Could you check a few things on this drawing? It's one solid part, dimensions in mm from its lowest x, y, z. A direction names the side the tool comes from. Round coordinates to 2 decimals unless told otherwise and drop trailing zeros. Loops run counter-clockwise (first coordinate to the right, second up) from the corner with the lowest first, then second, coordinate; pieces in that order, holes last. Notation, with made-up numbers: (79, 16) -> (106, 16) arc R27 cw to (106, 54) -> close; hole circle Ø5 at (83.25, 30.5). An arc over 180 degrees is marked (long way). Write each question's results on one line, items separated by ' | '.
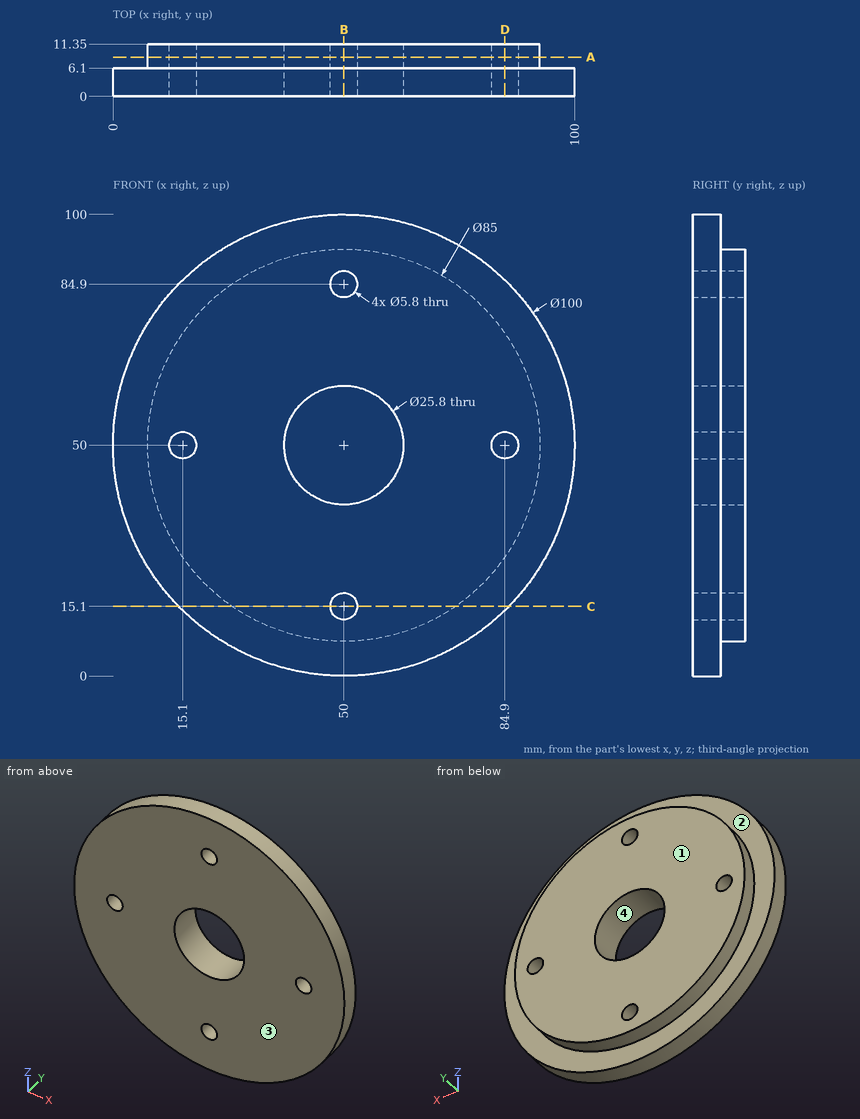
1) I need wall thicknesses on line 1 (X direction, y = 6.25, z = 50); line 2 (Z direction, x = 50, y = 4.5). Which ranges of each line are inside material? Lowest first, please.
Model answer:
line 1: x = 7.5 to 12.2, 18 to 37.1, 62.9 to 82, 87.8 to 92.5 | line 2: z = 0 to 12.2, 18 to 37.1, 62.9 to 82, 87.8 to 100
2) I'm going to push flat-ended pins straight in: pin 1 (3 mm diameter, centred on x = 40.5, z = 52.5, fed in from -Y); pin 2 (2 mm diameter, centred on x = 33.5, z = 51, fed in from -Y); pin 3 (2 mm diameter, centred on y = 2, z = 18.5, fed in from -X); pin 4 (6 mm diameter, centred on x = 38.5, y = 8.5, fed in from -Z). Where does each tip first touch, or does it pass through?
Model answer:
pin 1: passes through | pin 2: stops at y = 0 | pin 3: stops at x = 10.38 | pin 4: stops at z = 0.95
3) I want a section at C-C, the plane z = 15.1. Write out the boundary of the cut face in (x, y).
Model answer:
outline: (14.2, 0) -> (47.1, 0) -> (47.1, 11.35) -> (25.75, 11.35) -> (25.75, 6.1) -> (14.2, 6.1) -> close; (52.9, 0) -> (85.8, 0) -> (85.8, 6.1) -> (74.25, 6.1) -> (74.25, 11.35) -> (52.9, 11.35) -> close
4) I want a section at B-B, the plane x = 50. Write out the boundary of the cut face in (y, z), plus the area to 3 significant figures.
Model answer:
outline: (0, 0) -> (6.1, 0) -> (6.1, 7.5) -> (11.35, 7.5) -> (11.35, 12.2) -> (0, 12.2) -> close; (0, 18) -> (11.35, 18) -> (11.35, 37.1) -> (0, 37.1) -> close; (0, 62.9) -> (11.35, 62.9) -> (11.35, 82) -> (0, 82) -> close; (0, 87.8) -> (11.35, 87.8) -> (11.35, 92.5) -> (6.1, 92.5) -> (6.1, 100) -> (0, 100) -> close | area: 632 mm2
5) I want a section at D-D, the plane x = 84.9. Write out the boundary of the cut face in (y, z), plus the area to 3 significant figures.
Model answer:
outline: (0, 14.2) -> (6.1, 14.2) -> (6.1, 25.75) -> (11.35, 25.75) -> (11.35, 47.1) -> (0, 47.1) -> close; (0, 52.9) -> (11.35, 52.9) -> (11.35, 74.25) -> (6.1, 74.25) -> (6.1, 85.8) -> (0, 85.8) -> close | area: 626 mm2
6) I want a section at A-A, the plane y = 8.5. Write out the boundary of the cut face in (x, z).
Model answer:
outline: circle Ø85 at (50, 50); hole circle Ø5.8 at (15.1, 50); hole circle Ø25.8 at (50, 50); hole circle Ø5.8 at (50, 15.1); hole circle Ø5.8 at (50, 84.9); hole circle Ø5.8 at (84.9, 50)
7) For the marked faces 1 and 2, which set-ups out of +Z, -Z, +X, -X, +Y, -Y let a thin tool reach every point of the face, with its end or its side?
Model answer:
face 1: +Z, -Z, +X, -X, +Y | face 2: +Y
8) If we mould it in two halves opening along X, with no side actions, what happens to the marked faces 3 and 4? For each: released by +X, released by -X, zero draft, split by the parting line, or undercut.
Model answer:
face 3: zero draft | face 4: undercut
